Input: part model. Units: mm. Frame: model coordinates. Coordinates: 2 decimals unless noted, no trailing zeros. Loops run counter-clockwise (first coordinate to the right, second up) from the corner with the lowest first, then second, coordinate; pieces in that order, holes last. Notation, with made-up numbers: (39, 34.25) - (64, 34.25) arc R23 ccw to (64, 42.25) - close; hole circle Ø9 at (15, 73.5). An arc over 180 degrees is marked (long way). Use a Markdown table: item, result. Add a question column.
1. Contact query for flat-ended pins moving along their axis: P1, Ø2, axis at x = -2.5, y = 96.5, coming from the -Z side; P2, Ø1.2, axis at y = 2.5, z = 0, coming from the -X side; P3, Ø0.8, axis at x = 0.5, z = 0, coming from the -Y side; P4, Ø0.6, axis at y = 7.5, z = 0, coming from the -X side. Output: stop coordinate, or through.
2. Ray query, L1, parallel to Y at x = 0.8, z = 0; L2, parallel to Z at x = 0, y = 0.2 (3 decimals); L3, parallel to X at y = 0.4, z = 0. Return the intervals inside material, ascending. Write a range as [from, to].
3. Section query A-A on y = 60. Return the cut outline in (x, z), then the cut area to 3 significant figures.
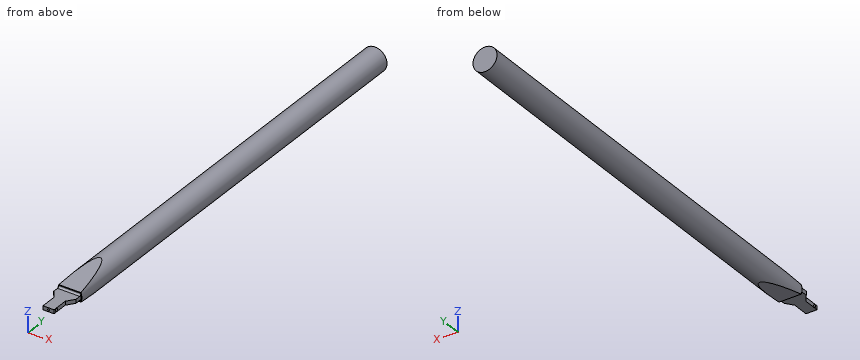
```python
from build123d import *

# Parameters (mm, degrees)
SKETCH1_W           = 3
SKETCH1_H           = 1.05
BOSS_EXTRUDE1_DEPTH = 2.4
SKETCH2_R           = 0.4
CUT_EXTRUDE1_DEPTH  = 3
SKETCH3_W           = 6
SKETCH3_H           = 2
SKETCH3_W_2         = 3
BOSS_EXTRUDE2_DEPTH = 1.05
CUT_EXTRUDE2_REACH  = 10.4
SKETCH4_R           = 0.25
SKETCH5_R           = 3.25
BOSS_EXTRUDE3_DEPTH = 120
FILLET2_R           = 0.5
CUT_EXTRUDE3_DEPTH  = 3.25


with BuildPart() as part:
    # Sketch1 → Boss-Extrude1 (new body)
    with BuildSketch(Plane(origin=(0, 0, 0), x_dir=(1, 0, 0), z_dir=(0, 1, 0))):
        Rectangle(SKETCH1_W, SKETCH1_H)
    extrude(amount=BOSS_EXTRUDE1_DEPTH)

    # Sketch2 → Cut-Extrude1 (cut)
    with BuildSketch(Plane(origin=(1.5, 0, 0), x_dir=(0, 0, -1), z_dir=(1, 0, 0))):
        with Locations((0, 0.9)):
            Circle(SKETCH2_R)
    extrude(amount=-CUT_EXTRUDE1_DEPTH, mode=Mode.SUBTRACT)

    # Sketch3 → Boss-Extrude2 (add)
    with BuildSketch(Plane.XY.offset(0.525)):
        with Locations((0, 7.4)):
            Rectangle(SKETCH3_W, SKETCH3_H)
        Polygon((3, 6.4), (1.5, 4.4), (-1.5, 4.4), (-3, 6.4), align=None)
        with Locations((0, 3.4)):
            Rectangle(SKETCH3_W_2, SKETCH3_H)
    extrude(amount=-BOSS_EXTRUDE2_DEPTH)

    # Sketch4 → Cut-Extrude2 (cut, up to next)
    with BuildSketch(Plane.XZ, mode=Mode.PRIVATE) as cut_extrude2_sk1:
        Circle(SKETCH4_R)
    cut_extrude2_tool1 = extrude(cut_extrude2_sk1.sketch, amount=-CUT_EXTRUDE2_REACH, mode=Mode.PRIVATE) & part.part
    add(cut_extrude2_tool1.solids().sort_by_distance((0, 0, 0))[0], mode=Mode.SUBTRACT)

    # Sketch5 → Boss-Extrude3 (add)
    with BuildSketch(Plane(origin=(0, 8.4, 0), x_dir=(1, 0, 0), z_dir=(0, 1, 0))):
        Circle(SKETCH5_R)
    extrude(amount=BOSS_EXTRUDE3_DEPTH)

    # Fillet2
    fillet2_edges = [part.edges().sort_by_distance(p)[0] for p in [
        (0, 8.4, -0.525),
        (0, 8.4, 0.525),
    ]]
    fillet(fillet2_edges, radius=FILLET2_R)

    # Sketch6 → Cut-Extrude3 (cut, symmetric)
    with BuildSketch(Plane(origin=(0, 0, 0), x_dir=(0, 0, -1), z_dir=(1, 0, 0))):
        Polygon((-3.25, 8.4), (-3.25, 20.4), (-1.25, 8.4), align=None)
        Polygon((3.25, 8.4), (3.25, 20.4), (1.25, 8.4), align=None)
    extrude(amount=CUT_EXTRUDE3_DEPTH, both=True, mode=Mode.SUBTRACT)


solid = part.part
```
Resolved:
| question | item | result |
|---|---|---|
| 1 | P1 | z = -2.88 |
| 1 | P2 | x = -1.5 |
| 1 | P3 | y = 0 |
| 1 | P4 | x = -3 |
| 2 | L1 | [0, 0.5], [1.3, 128.4] |
| 2 | L2 | [-0.525, -0.25], [0.25, 0.525] |
| 2 | L3 | [-1.5, -0.25], [0.25, 1.5] |
| 3 | outline | circle Ø6.5 at (0, 0) |
| 3 | area | 33.2 mm² |
